Design review of the part built by this model. Coordinates are the model's own, in mm. A direction names the side the tool comes from. Give positions to 0.01 mm unless a question says otherwise; leave off trailing zeros. Write each loop counter-clockwise with the first axis right and the second up, starting at its lowest first coordinate (ties: lowest second). Pieces come first, ordered by that corner, then holes. Notation, with made-up numbers: (-16, 81) -> (2, 81) arc R26 cw to (2, 111) -> close; hole circle Ø3 at (-40, -34.75). An arc over 180 degrees is marked (long way). Answer as a JSON object with one key per item and string values.
```python
from build123d import *

# Parameters (mm, degrees)
F1_DEPTH = 3
F3_D     = 4


# Not quite as in the source:
# - a feature names something its author has since deleted; it is built from what else it names


with BuildPart() as f1:
    # F0 (on Top) → F1 (new body)
    with BuildSketch(Plane.XY):
        with BuildLine():
            Line((14.0881506171, 0), (14.0881506171, 3.5))
            ThreePointArc((14.0881506171, 3.5), (7.9876115371, 4.4807007673), (1.8788639221, 3.5525016304))
            ThreePointArc((1.8788639221, 3.5525016304), (2.1302987541, 2.666794093), (2.2150684857, 1.75))
            ThreePointArc((2.2150684857, 1.75), (2.1302987541, 0.833205907), (1.8788639221, -0.0525016304))
            ThreePointArc((1.8788639221, -0.0525016304), (7.9876115371, -0.9807007673), (14.0881506171, 0))
        make_face()
        with BuildLine():
            Line((21.6484292713, 3.5), (21.6484292713, 0))
            Line((21.6484292713, 0), (27.6484292713, 0))
            ThreePointArc((27.6484292713, 0), (29.3682210792, -0.4835632197), (30.5839958787, -1.7925356741))
            Line((30.5839958787, -1.7925356741), (50.5839958787, -1.7925356741))
            Line((50.5839958787, -1.7925356741), (58.9184745012, 10.6788903105))
            Line((58.9184745012, 10.6788903105), (50.5839958787, 3.5))
            ThreePointArc((50.5839958787, 3.5), (42.7439688076, 1.4762635236), (34.9039417364, 3.5))
            Line((34.9039417364, 3.5), (21.6484292713, 3.5))
        make_face()
        with BuildLine():
            Line((16.0120092332, 2.9430498835), (14.0881506171, 3.5))
            Line((14.0881506171, 3.5), (14.0881506171, 0))
            Line((14.0881506171, 0), (16.0120092332, 0))
            Line((16.0120092332, 0), (16.0120092332, -4.25))
            Line((16.0120092332, -4.25), (15.1717471866, -6.6045614651))
            Line((15.1717471866, -6.6045614651), (25.9923258961, -11.7925356741))
            Line((25.9923258961, -11.7925356741), (25.9923258961, -1.7925356741))
            ThreePointArc((25.9923258961, -1.7925356741), (24.192277602, -3.6786508222), (21.6484292713, -4.25))
            Line((21.6484292713, -4.25), (21.6484292713, 0))
            Line((21.6484292713, 0), (21.6484292713, 3.5))
            Line((21.6484292713, 3.5), (21.6484292713, 5.75))
            ThreePointArc((21.6484292713, 5.75), (22.2690927393, 6.6798640271), (23.1717471866, 7.3394739101))
            ThreePointArc((23.1717471866, 7.3394739101), (23.3522374925, 6.5091821103), (23.1717471866, 5.6788903105))
            ThreePointArc((23.1717471866, 5.6788903105), (25.6717471866, 8.1788903105), (23.1717471866, 10.6788903105))
            Line((23.1717471866, 10.6788903105), (15.1717471866, 10.6788903105))
            Line((15.1717471866, 10.6788903105), (16.0120092332, 5.75))
            Line((16.0120092332, 5.75), (16.0120092332, 2.9430498835))
        make_face()
        with BuildLine():
            ThreePointArc((1.7150684857, 3.5), (1.7969097631, 3.5264269002), (1.8788639221, 3.5525016304))
            ThreePointArc((1.8788639221, 3.5525016304), (-7.7849315143, 1.75), (1.8788639221, -0.0525016304))
            ThreePointArc((1.8788639221, -0.0525016304), (1.7969097631, -0.0264269002), (1.7150684857, 0))
            Line((1.7150684857, 0), (1.7150684857, 1.75))
            Line((1.7150684857, 1.75), (1.7150684857, 3.5))
        make_face()
        with BuildLine():
            ThreePointArc((2.2150684857, 1.75), (2.1302987541, 2.666794093), (1.8788639221, 3.5525016304))
            ThreePointArc((1.8788639221, 3.5525016304), (1.7969097631, 3.5264269002), (1.7150684857, 3.5))
            Line((1.7150684857, 3.5), (1.7150684857, 1.75))
            Line((1.7150684857, 1.75), (2.2150684857, 1.75))
        make_face()
        with BuildLine():
            ThreePointArc((1.8788639221, -0.0525016304), (2.1302987541, 0.833205907), (2.2150684857, 1.75))
            Line((2.2150684857, 1.75), (1.7150684857, 1.75))
            Line((1.7150684857, 1.75), (1.7150684857, 0))
            ThreePointArc((1.7150684857, 0), (1.7969097631, -0.0264269002), (1.8788639221, -0.0525016304))
        make_face()
    extrude(amount=F1_DEPTH)

    # F3 (through all)
    with Locations(Plane.XY.offset(3)):
        with Locations((-3.7849315143, 1.7499999964)):
            Hole(F3_D / 2)


solid = f1.part
```
(1) For line 1 along X through (y, z) = (-2.5, 2.05); line 2 along X through (y, z) = (-2.25, 2); line 3 along Y through (x, z) = (32.5, 2.1), list the stretches that pass through material, from the lowest coordinate up.
Here are the results:
{"line 1": "x = -5.42 to -0.15, 16.01 to 21.65, 25.55 to 25.99", "line 2": "x = -5.78 to 0.22, 16.01 to 21.65, 25.73 to 25.99", "line 3": "y = -1.79 to 3.5"}
(2) For faces 1 (the cylindrical face through (24.224, -3.66, 1.479)), 2 (the flat face through (25.992, -7, 1)), 3 (the flat face through (54.81, 7.14, 1.48)), 4 (the flat face through (15.6, -5.4, 1.5)), 5 (the cylindrical face through (29.347, -0.47, 1.479)), list the 3-axis set-ups (+Z, -Z, +X, -X, +Y, -Y) from which the entire face can be reached by the end or side of a thin tool; tool diameter is ignored.
Here are the results:
{"face 1": "+Z, -Z", "face 2": "+Z, -Z, +X, -Y", "face 3": "+Z, -Z, +Y", "face 4": "+Z, -Z, -X", "face 5": "+Z, -Z, -Y"}
(3) We need section C-C, the plane y = -5. State the section outline as (x, z) points, then the cut area to 3 significant figures.
Here are the results:
{"outline": "(15.74, 0) -> (25.99, 0) -> (25.99, 3) -> (15.74, 3) -> close", "area": "30.7 mm²"}
(4) Clearance check with flat-ended pins moving along their axes: pin 1 (1 mm diameter, centred on x = 52, y = 6, fed in from +Z); pin 2 (1 mm diameter, centred on x = 13.5, z = 1.5, fed in from -Y); pin 3 (1.5 mm diameter, centred on x = 28.5, z = 1, fed in from +Y); pin 4 (1.5 mm diameter, centred on y = -3, z = 1.5, fed in from +X). State where each tip first meets the part, or that it passes through.
Here are the results:
{"pin 1": "passes through", "pin 2": "stops at y = -0.32", "pin 3": "stops at y = 3.5", "pin 4": "stops at x = 25.99"}
(5) The part is to be moulded in two halves that separate along Y. For faces 6 (the cylindrical face through (-5.693, 2.351, 1.479)), 7 (the cylindrical face through (8.07, 4.48, 1.48)), 8 (the flat face through (54.693, 4.356, 1.479)), say which applies: +Y half, -Y half, draft (parallel to the pull), parting line (faces both ways), or undercut.
Here are the results:
{"face 6": "undercut", "face 7": "+Y half", "face 8": "-Y half"}
(6) We need section B-B, the plane x = 32.5. State the section outline as (y, z) points, then the cut area to 3 significant figures.
Here are the results:
{"outline": "(-1.79, 0) -> (3.5, 0) -> (3.5, 3) -> (-1.79, 3) -> close", "area": "15.9 mm²"}
(7) We need section A-A, the plane z = 1.15. State the section outline as (x, y) points.
Here are the results:
{"outline": "(1.88, -0.05) arc R20 ccw to (14.09, 0) -> (16.01, 0) -> (16.01, -4.25) -> (15.17, -6.6) -> (25.99, -11.79) -> (25.99, -1.79) arc R4.5 cw to (21.65, -4.25) -> (21.65, 0) -> (27.65, 0) arc R3.3 cw to (30.58, -1.79) -> (50.58, -1.79) -> (58.92, 10.68) -> (50.58, 3.5) arc R16.2 cw to (34.9, 3.5) -> (21.65, 3.5) -> (21.65, 5.75) arc R3.2 cw to (23.17, 7.34) arc R2 cw to (23.17, 5.68) arc R2.5 ccw to (23.17, 10.68) -> (15.17, 10.68) -> (16.01, 5.75) -> (16.01, 2.94) -> (14.09, 3.5) arc R20 ccw to (1.88, 3.55) arc R5 ccw (long way) to start; hole circle Ø4 at (-3.78, 1.75)"}
